```python
from build123d import *

# Parameters (mm, degrees)
SKETCH1_R           = 3.2639
BOSS_EXTRUDE1_DEPTH = 3.175
FILLET2_R           = 4.7625
SKETCH3_R           = 3.2639
CUT_EXTRUDE1_DEPTH  = 3.175


with BuildPart() as part:
    # Sketch1 → Boss-Extrude1 (new body)
    with BuildSketch(Plane(origin=(0, 0, 0), x_dir=(0, 0, -1), z_dir=(1, 0, 0))):
        Polygon((182.388740953, 7.963264406), (181.834774733, 20.65117682), (171.980710149, 20.220939069), (173.069858002, -4.724648008), (182.942707172, -4.724648008), align=None)
        with Locations((177.123417321, 15.496291061)):
            Circle(SKETCH1_R, mode=Mode.SUBTRACT)
        with Locations((177.8, 0)):
            Circle(SKETCH1_R, mode=Mode.SUBTRACT)
    extrude(amount=BOSS_EXTRUDE1_DEPTH)

    # Fillet2
    fillet2_edges = [part.edges().sort_by_distance(p)[0] for p in [
        (1.5875, -4.724648008, -182.942707172),
        (1.5875, -4.724648008, -173.069858002),
        (1.5875, 20.220939069, -171.980710149),
        (1.5875, 20.65117682, -181.834774733),
    ]]
    fillet(fillet2_edges, radius=FILLET2_R)

    # Sketch3 → Cut-Extrude1 (cut)
    with BuildSketch(Plane(origin=(0, 7.963264406, -182.388740953), x_dir=(-1, 0, 0), z_dir=(0, 0.04361938736533578, -0.9990482215818579))):
        with Locations((0.79375, 0.106236202)):
            Circle(SKETCH3_R)
    extrude(amount=-CUT_EXTRUDE1_DEPTH, mode=Mode.SUBTRACT)


solid = part.part
```
The listing builds one solid part. Answer for the finished solid, in the listing's coordinates (mm). Give positions to 0.01 mm unless a question says otherwise; leave off trailing zeros. Order: outer loops, then holes, each group sorted by start corner. A loop starts at its lowest first (then second) coordinate and runs counter-clockwise, first axis right, second up.
Item 1: The part is cut by section B-B, the plane x = 0.6. Count the separate pieces of the cut face and the enclosed holes in it, and give its area (3 significant figures).
From the geometry:
separate pieces: 1
enclosed holes: 2
area: 143 mm2
Item 2: Find the intervals of material crossed by probe 1 along Y at (x, z) = (2.7, -179.25); probe 2 along Y at (x, z) = (0.35, -177.75); probe 3 along Y at (x, z) = (1.85, -179.5), in increasing order.
From the geometry:
probe 1: y = -4.55 to -2.92, 2.92 to 13.02, 17.97 to 20.02
probe 2: y = -4.72 to -3.26, 3.26 to 12.29, 18.7 to 20.43
probe 3: y = -4.47 to -2.79, 2.79 to 6.03, 9.86 to 13.26, 17.73 to 19.9
Item 3: The part is cut by section A-A, the plane y = -0.75. Give the vertices of the cut face in (x, z) (3 decimals).
From the geometry:
outline: (0, -182.665) - (3.175, -182.665) - (3.175, -180.977) - (0, -180.977) - close; (0, -174.623) - (3.175, -174.623) - (3.175, -172.932) - (0, -172.932) - close
Item 4: For a pull along Z with two mould halves and no side action, classify faces 1 (the face through (1.61, -3.22, -181.44)), 2 (the face through (1.57, 14.25, -180.14)), 3 (the face through (3.175, 8, -177)) as pulls with the +Z half, pulls with the -Z half, needs draft (parallel to the pull), parting line crosses it, or undercut.
From the geometry:
face 1: pulls with the -Z half
face 2: undercut
face 3: needs draft
Item 5: The part is cut by section C-C, the plane y = 16.5. Give the vertices of the cut face in (x, z) (3 decimals), and give its area (3 significant figures).
From the geometry:
outline: (0, -181.977) - (3.175, -181.977) - (3.175, -180.229) - (0, -180.229) - close; (0, -174.018) - (3.175, -174.018) - (3.175, -172.257) - (0, -172.257) - close
area: 11.1 mm2
Item 6: Given pin 1 Ø4 at (y, z) = (15.5, -177.12) entering from +X; pin 2 Ø1 at (x, z) = (1.5, -176.5) entering from +Y, each flat-ended and moving along its own axis, determine where each tip first touches the part or whether it passes through.
From the geometry:
pin 1: passes through
pin 2: stops at y = 20.44
